Geometry: see drawing. Coordinates: mm, zero at the bounding-box minimum. A direction names the side the tool comes from. Round coordinates to 2 decimals unless told otherwise and drop trailing zeros. Loops run counter-clockwise (first coordinate to the right, second up) from the corner with the lowest first, then second, coordinate; pieces in that order, holes last.
(1) Section C-C, the plane z = 45. Return the cut outline in (x, y).
(2) Material intervals for probe 1 along Y at (x, z) = (33.6, 12.5); probe 2 along X at (y, z) = (8, 34); probe 3 along Y at (x, z) = (7, 7), sorted ascending.
(3) Section A-A, the plane z = 52.5. Return the cut outline in (x, y).
(4) First-contact query: pin 1 Ø12 at (x, y) = (25, 65) entering from -Z. Flat tip, straight axial feed; report the tip coordinate or a pass-through.
(5) Section B-B, the plane x = 8.5. Return the cut outline in (y, z).
(6) Set-up query: the marked faces 1 and 2. Return all of +Z, -Z, +X, -X, +Y, -Y with unobstructed straight access to the full face (end or side cutting, diameter ignored); none if empty.
(7) Section D-D, the plane y = 40. Return the cut outline in (x, z).
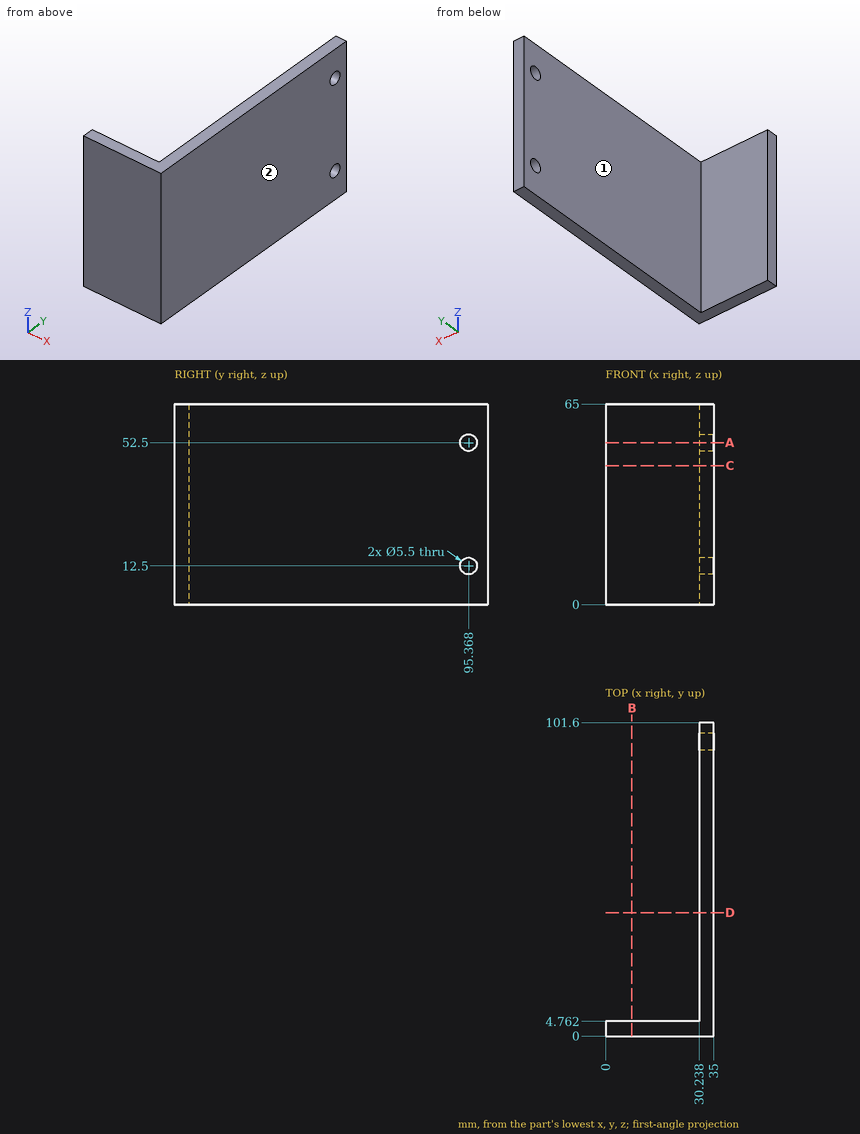
Output values:
1. outline: (0, 0) - (35, 0) - (35, 101.6) - (30.24, 101.6) - (30.24, 4.76) - (0, 4.76) - close
2. probe 1: y = 0 to 92.62, 98.12 to 101.6
2. probe 2: x = 30.24 to 35
2. probe 3: y = 0 to 4.76
3. outline: (0, 0) - (35, 0) - (35, 92.62) - (30.24, 92.62) - (30.24, 4.76) - (0, 4.76) - close; (30.24, 98.12) - (35, 98.12) - (35, 101.6) - (30.24, 101.6) - close
4. pin 1: stops at z = 0
5. outline: (0, 0) - (4.76, 0) - (4.76, 65) - (0, 65) - close
6. face 1: +Z, -Z, -X, +Y
6. face 2: +Z, -Z, +X, +Y, -Y
7. outline: (30.24, 0) - (35, 0) - (35, 65) - (30.24, 65) - close
